Geometry: final body of the model. Coordinates: model frame, mm. A direction names the side the tool comes from. Give positions to 0.01 mm unless a question says otherwise; leave off trailing zeros. Loops run counter-clockwise (first coordinate to the right, second up) from the corner with the lowest first, then second, coordinate; pieces in that order, holes last.
1. Section A-A, the plane x = 100. Output: boundary loops of the cut face in (y, z), then the cut area to 3 significant figures.
2. Section C-C, the plane y = 44. Output: boundary loops of the cut face in (x, z), then the cut area to 3 significant figures.
3. Section B-B, the plane z = 1.1. State how many separate pieces and enclosed holes the cut face has, then the cut area to 3 significant figures.
4. Section D-D, the plane x = 32. Output: boundary loops of the cut face in (y, z), then the cut area to 3 significant figures.
5. Access query for faces 4 (the face through (2, 2.1, 2)), 5 (the face through (111, 50, 2)). Directions: +Z, -Z, +X, -X, +Y, -Y. A direction counts if a zero-diameter tool reaches every point of the face in a straight line with its end or side. Return the directions, or none.
6. Draft query along Y for faces 1 (the face through (13, 50, 2)), 2 (the face through (121.9, 82, 2)), 3 (the face through (61, 24, 4)). Return one class per face: +Y half, -Y half, draft (parallel to the pull), parting line (faces both ways), or undercut.
7. First-contact query: P1, Ø2.5, axis at x = 7, y = 77, coming from the +Z side. Flat tip, straight axial feed; report the tip coordinate or a pass-through.
8. Material intervals for line 1 along Y through (x, z) = (117, 3.1); line 2 along Y through (x, z) = (92, 1); line 3 along X through (y, z) = (65, 0.75), sorted ascending.
from build123d import *

# Parameters (mm, degrees)
CROQUIS1_W              = 124
CROQUIS1_H              = 84
CROQUIS1_R              = 2
CROQUIS1_R_2            = 4
CROQUIS1_W_2            = 98
CROQUIS1_H_2            = 40
SALIENTE_EXTRUIR1_DEPTH = 4
REDONDEO1_R             = 7


with BuildPart() as part:
    # Croquis1 → Saliente-Extruir1 (new body)
    with BuildSketch(Plane.XY):
        with Locations((62, 42)):
            Rectangle(CROQUIS1_W, CROQUIS1_H)
        with Locations((7, 77)):
            Circle(CROQUIS1_R, mode=Mode.SUBTRACT)
        with Locations((117, 77)):
            Circle(CROQUIS1_R, mode=Mode.SUBTRACT)
        with Locations((117, 7)):
            Circle(CROQUIS1_R, mode=Mode.SUBTRACT)
        with Locations((7, 7)):
            Circle(CROQUIS1_R, mode=Mode.SUBTRACT)
        with Locations((32, 12)):
            Circle(CROQUIS1_R_2, mode=Mode.SUBTRACT)
        with Locations((62, 12)):
            Circle(CROQUIS1_R_2, mode=Mode.SUBTRACT)
        with Locations((92, 12)):
            Circle(CROQUIS1_R_2, mode=Mode.SUBTRACT)
        with Locations((62, 50)):
            Rectangle(CROQUIS1_W_2, CROQUIS1_H_2, mode=Mode.SUBTRACT)
    extrude(amount=SALIENTE_EXTRUIR1_DEPTH)

    # Redondeo1
    redondeo1_edges = [part.edges().sort_by_distance(p)[0] for p in [
        (0, 84, 2),
        (124, 84, 2),
        (124, 0, 2),
        (0, 0, 2),
    ]]
    fillet(redondeo1_edges, radius=REDONDEO1_R)


solid = part.part
Answers below:
1. outline: (0, 0) - (30, 0) - (30, 4) - (0, 4) - close; (70, 0) - (84, 0) - (84, 4) - (70, 4) - close
1. area: 176 mm2
2. outline: (0, 0) - (13, 0) - (13, 4) - (0, 4) - close; (111, 0) - (124, 0) - (124, 4) - (111, 4) - close
2. area: 104 mm2
3. separate pieces: 1
3. enclosed holes: 8
3. area: 6,250 mm2
4. outline: (0, 0) - (8, 0) - (8, 4) - (0, 4) - close; (16, 0) - (30, 0) - (30, 4) - (16, 4) - close; (70, 0) - (84, 0) - (84, 4) - (70, 4) - close
4. area: 144 mm2
5. face 4: +Z, -Z, -X, -Y
5. face 5: +Z, -Z
6. face 1: undercut
6. face 2: +Y half
6. face 3: draft
7. P1: passes through
8. line 1: y = 0 to 5, 9 to 75, 79 to 84
8. line 2: y = 0 to 8, 16 to 30, 70 to 84
8. line 3: x = 0 to 13, 111 to 124
